Can you work these out from the model? Positions are in its coordinate system, mm. Face numbers are marked on the shaded views. Round coordinates to 2 decimals unless told otherwise and drop trailing zeros. Loops run counter-clockwise (first coordinate to the right, second up) from the corner with the lowest first, then second, coordinate; pieces in that order, holes last.
(1) I want a section at C-C on x = -5.5. Write out the boundary of the cut face in (y, z), plus the area to 3 significant figures.
(2) I want a section at A-A on y = -26. Write out the boundary of the cut face in (x, z), plus the area to 3 significant figures.
(3) I want a section at B-B on z = -7.5. Write out the boundary of the cut face in (x, y), plus the area to 3 significant figures.
(4) I want a section at D-D on y = -3. Write out the boundary of the cut face in (x, z).
(5) Thinking about a two-plate mould opening in Z: for the marked faces 1, 2 and 3, which applies, released by +Z, released by -Z, zero draft, split by the parting line, or undercut?
(6) If I drill on line 1 along Y through (x, z) = (-26, -41); line 2 along Z through (x, y) = (-24, -15); line 3 along X through (y, z) = (-34, -23), over which ranges is the centre line in solid material (lowest first)?
(7) Will these pins go through, and if not, where does the flat tip stop? pin 1 Ø12 at (y, z) = (-17, -26) entering from +X; pin 2 Ø1 at (y, z) = (-15, -20.5) entering from +X; pin 3 Ø12 at (y, z) = (-23, -26.5) entering from +X.
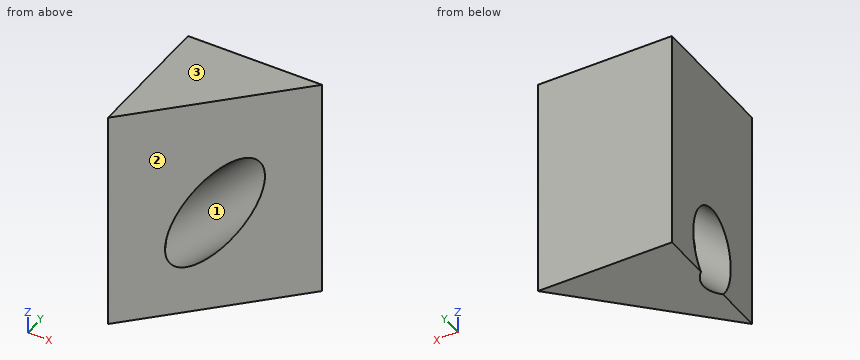
from build123d import *

# Parameters (mm, degrees)
F0_W          = 38.1
F0_H          = 63.5
F1_DEPTH      = 38.1
F4_R          = 8.89
F5_DEPTH      = 50.8
F5_DEPTH_BACK = 76.2
F7_DEPTH      = 76.2


with BuildPart() as f1:
    # F0 (on Front) → F1 (new body)
    with BuildSketch(Plane.XZ):
        with Locations((-19.05, -31.75)):
            Rectangle(F0_W, F0_H)
    extrude(amount=F1_DEPTH)

    # F4 (on line) → F5 (cut, two sides)
    with BuildSketch(Plane(origin=(-7.62, 0, -7.62), x_dir=(0.7071067812, 0, -0.7071067812), z_dir=(-0.7071067812, 0, -0.7071067812))) as f5_sk:
        with Locations((10.7763073453, 19.05)):
            Circle(F4_R)
    extrude(amount=-F5_DEPTH, mode=Mode.SUBTRACT)
    extrude(f5_sk.sketch, amount=F5_DEPTH_BACK, mode=Mode.SUBTRACT)

    # F6 (on face) → F7 (cut)
    with BuildSketch(Plane.XY):
        Polygon((0, -38.1), (0, 0), (-38.1, -38.1), align=None)
    extrude(amount=-F7_DEPTH, mode=Mode.SUBTRACT)


solid = f1.part
Filled sheet:
1. outline: (-5.5, -63.5) - (0, -63.5) - (0, 0) - (-5.5, 0) - close
1. area: 349 mm2
2. outline: (-38.1, -63.5) - (-26, -63.5) - (-26, -49.08) - (-38.1, -61.18) - close; (-38.1, -45.5) - (-26, -33.4) - (-26, 0) - (-38.1, 0) - close
2. area: 579 mm2
3. outline: (-38.1, -38.1) - (0, 0) - (-38.1, 0) - close
3. area: 726 mm2
4. outline: (-38.1, -63.5) - (-3, -63.5) - (-3, 0) - (-38.1, 0) - close
5. face 1: undercut
5. face 2: zero draft
5. face 3: released by +Z
6. line 1: y = -10.16 to 0
6. line 2: z = -63.5 to -50.43, -28.05 to 0
6. line 3: x = -38.1 to -34
7. pin 1: stops at x = -15
7. pin 2: stops at x = -15.82
7. pin 3: stops at x = -19.19
